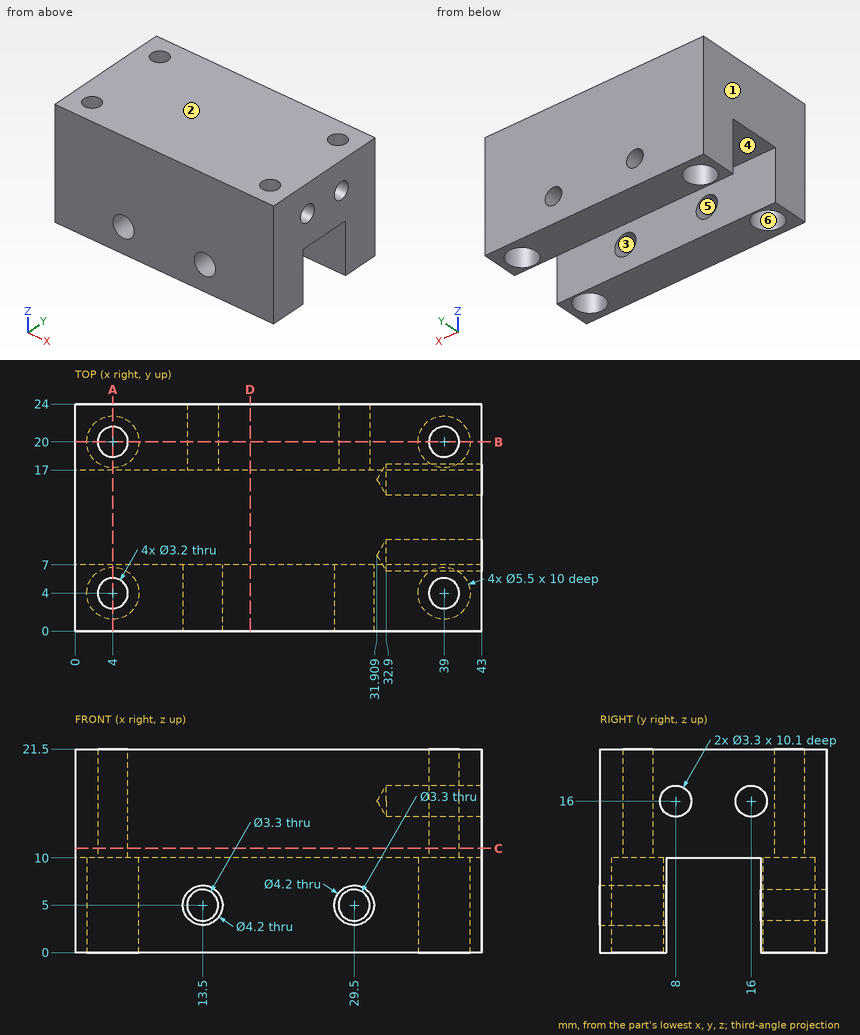
Source: three-view drawing plus pictorial views. Frame: mm from the lowest corner of the part. A direction names the side the tool comes from. Round coordinates to 2 decimals unless told otherwise and drop trailing zeros. Write each loop counter-clockwise with the first axis right and the second up, starting at its lowest first coordinate (ties: lowest second). Pieces come first, ordered by that corner, then holes. Notation, with made-up numbers: M 78,-15 L 102,-15 A26 ccw 102,5 Z; hole C 65.25,-32.75 d9. An arc over 180 degrees is marked long. One line per item, written item: value. Start each with the question number.
Item 1: Set-up query: the marked faces 4, 5 and 6. Return all of +Z, -Z, +X, -X, +Y, -Y with unobstructed straight access to the full face (end or side cutting, diameter ignored); none if empty.
Item 2: Ray query, L1, parallel to Y at x = 39, z = 3; L2, parallel to X at y = 4.25, z = 7.5; L3, parallel to X at y = 5.25, z = 4.5. Return the intervals inside material, ascending. Write a range as from..to.
Item 3: Section query D-D (x = 18.5). Return the cut outline in (y, z).
Item 4: Mould query, pull axis Z, two halves, no side actions, for the marked faces 1, 2 and 3. Classes: pulls with the +Z half, pulls with the -Z half, needs draft (parallel to the pull), parting line crosses it, or undercut.
Item 5: Pin query (flat end, axial travel): pin 1 (3 mm diameter, centred on x = 4.5, y = 5, fed in from -Z). Return the tip coordinate at first contact, or that it passes through.
Item 6: Section query B-B (y = 20). Return the cut outline in (x, z), plus the area to 3 significant figures.
Item 7: Section query A-A (x = 4). Return the cut outline in (y, z).
Item 8: Section query C-C (z = 11). Return the cut outline in (x, y).
Result set:
1. face 4: -Z, +X, -X
1. face 5: -Y
1. face 6: -Z
2. L1: y = 0..1.25, 6.75..7, 17..17.25, 22.75..24
2. L2: x = 0..1.26, 6.74..36.26, 41.74..43
2. L3: x = 0..1.55, 6.45..11.46, 15.54..27.46, 31.54..36.55, 41.45..43
3. outline: M 0,0 L 7,0 L 7,10 L 17,10 L 17,0 L 24,0 L 24,21.5 L 0,21.5 Z
4. face 1: needs draft
4. face 2: pulls with the +Z half
4. face 3: undercut
5. pin 1: stops at z = 10
6. outline: M 0,0 L 1.25,0 L 1.25,10 L 2.4,10 L 2.4,21.5 L 0,21.5 Z; M 5.6,10 L 6.75,10 L 6.75,0 L 36.25,0 L 36.25,10 L 37.4,10 L 37.4,21.5 L 5.6,21.5 Z; M 40.6,10 L 41.75,10 L 41.75,0 L 43,0 L 43,21.5 L 40.6,21.5 Z; hole C 13.5,5 d3.3; hole C 29.5,5 d3.3
6. area: 724 mm²
7. outline: M 0,0 L 1.25,0 L 1.25,10 L 2.4,10 L 2.4,21.5 L 0,21.5 Z; M 5.6,10 L 6.75,10 L 6.75,0 L 7,0 L 7,10 L 17,10 L 17,0 L 17.25,0 L 17.25,10 L 18.4,10 L 18.4,21.5 L 5.6,21.5 Z; M 21.6,10 L 22.75,10 L 22.75,0 L 24,0 L 24,21.5 L 21.6,21.5 Z
8. outline: M 0,0 L 43,0 L 43,24 L 0,24 Z; hole C 4,4 d3.2; hole C 4,20 d3.2; hole C 39,4 d3.2; hole C 39,20 d3.2
